```python
from build123d import *

# Parameters (mm, degrees)
SKETCH1_W           = 210
SKETCH1_H           = 450
SKETCH1_R           = 10
BOSS_EXTRUDE1_DEPTH = 6
SKETCH3_W           = 6
SKETCH3_H           = 24
BOSS_EXTRUDE3_DEPTH = 6
SKETCH2_W           = 24
SKETCH2_H           = 6
BOSS_EXTRUDE4_DEPTH = 6


with BuildPart() as part:
    # Sketch1 → Boss-Extrude1 (new body)
    with BuildSketch(Plane(origin=(0, 0, 0), x_dir=(1, 0, 0), z_dir=(0, 1, 0))):
        Rectangle(SKETCH1_W, SKETCH1_H)
        with Locations((0, -165)):
            Circle(SKETCH1_R, mode=Mode.SUBTRACT)
    extrude(amount=BOSS_EXTRUDE1_DEPTH)

    # Sketch3 → Boss-Extrude3 (add)
    with BuildSketch(Plane(origin=(0, 6, 0), x_dir=(1, 0, 0), z_dir=(0, 1, 0))):
        with Locations((-108, 192)):
            Rectangle(SKETCH3_W, SKETCH3_H)
        with Locations((108, 192)):
            Rectangle(SKETCH3_W, SKETCH3_H)
        with Locations((108, 144)):
            Rectangle(SKETCH3_W, SKETCH3_H)
        with Locations((108, 96)):
            Rectangle(SKETCH3_W, SKETCH3_H)
        with Locations((108, 48)):
            Rectangle(SKETCH3_W, SKETCH3_H)
        with Locations((108, 0)):
            Rectangle(SKETCH3_W, SKETCH3_H)
        with Locations((108, -48)):
            Rectangle(SKETCH3_W, SKETCH3_H)
        with Locations((108, -96)):
            Rectangle(SKETCH3_W, SKETCH3_H)
        with Locations((108, -144)):
            Rectangle(SKETCH3_W, SKETCH3_H)
        with Locations((108, -192)):
            Rectangle(SKETCH3_W, SKETCH3_H)
        with Locations((-108, 144)):
            Rectangle(SKETCH3_W, SKETCH3_H)
        with Locations((-108, 96)):
            Rectangle(SKETCH3_W, SKETCH3_H)
        with Locations((-108, 48)):
            Rectangle(SKETCH3_W, SKETCH3_H)
        with Locations((-108, 0)):
            Rectangle(SKETCH3_W, SKETCH3_H)
        with Locations((-108, -48)):
            Rectangle(SKETCH3_W, SKETCH3_H)
        with Locations((-108, -96)):
            Rectangle(SKETCH3_W, SKETCH3_H)
        with Locations((-108, -144)):
            Rectangle(SKETCH3_W, SKETCH3_H)
        with Locations((-108, -192)):
            Rectangle(SKETCH3_W, SKETCH3_H)
    extrude(amount=-BOSS_EXTRUDE3_DEPTH)

    # Sketch2 → Boss-Extrude4 (add)
    with BuildSketch(Plane(origin=(0, 6, 0), x_dir=(1, 0, 0), z_dir=(0, 1, 0))):
        with Locations((-72, 228)):
            Rectangle(SKETCH2_W, SKETCH2_H)
        with Locations((-24, 228)):
            Rectangle(SKETCH2_W, SKETCH2_H)
        with Locations((24, 228)):
            Rectangle(SKETCH2_W, SKETCH2_H)
        with Locations((72, 228)):
            Rectangle(SKETCH2_W, SKETCH2_H)
        with Locations((-72, -228)):
            Rectangle(SKETCH2_W, SKETCH2_H)
        with Locations((-24, -228)):
            Rectangle(SKETCH2_W, SKETCH2_H)
        with Locations((24, -228)):
            Rectangle(SKETCH2_W, SKETCH2_H)
        with Locations((72, -228)):
            Rectangle(SKETCH2_W, SKETCH2_H)
    extrude(amount=-BOSS_EXTRUDE4_DEPTH)


solid = part.part
```
Part model, mm, in its own coordinate system. Round coordinates to 2 decimals unless told otherwise and drop trailing zeros. Loops run counter-clockwise (first coordinate to the right, second up) from the corner with the lowest first, then second, coordinate; pieces in that order, holes last.
Item 1: Cut at B-B, the plane z = 165. Give the cut face in (x, y).
Item 2: Drop flat-ended pins along their axis: P1, Ø1.8, axis at x = 109, y = 3.5, coming from the -Z side; P2, Ø1.8, axis at x = -108, y = 3.5, coming from the +Z side; P3, Ø1.8, axis at y = 4.5, z = 21.5, coming from the -X side. Give the stop position or say it passes through.
Item 3: Cut at A-A, the plane x = 0. Give the cut face in (y, z).
Item 4: Drill centre lines: line 1 (Z direction, x = 0, y = 3.4); line 2 (X direction, y = 3.05, z = 165); line 3 (X direction, y = 5.3, z = 166). Where is each one in solid material? Low to high.
Item 5: Cut at C-C, the plane x = -89. Give the cut face in (y, z).
Item 6: Mould opens along X. For faces 1 (the face through (-2, 6, -3)), 2 (the face through (-2.17, 2.96, 174.76)) say: +X half, -X half, draft (parallel to the pull), parting line (faces both ways), or undercut.
A:
1. outline: (-105, 0) - (-10, 0) - (-10, 6) - (-105, 6) - close; (10, 0) - (105, 0) - (105, 6) - (10, 6) - close
2. P1: stops at z = -204
2. P2: stops at z = 204
2. P3: stops at x = -105
3. outline: (0, -225) - (6, -225) - (6, 155) - (0, 155) - close; (0, 175) - (6, 175) - (6, 225) - (0, 225) - close
4. line 1: z = -225 to 155, 175 to 225
4. line 2: x = -105 to -10, 10 to 105
4. line 3: x = -105 to -9.95, 9.95 to 105
5. outline: (0, -225) - (6, -225) - (6, 225) - (0, 225) - close
6. face 1: draft
6. face 2: undercut
